For this review, use the dimensioned drawing (mm, ordinates from the lowest corner) and the shaded views. Round coordinates to 2 decimals unless told otherwise and drop trailing zeros. Order: outer loops, then holes, each group sorted by start corner. A loop starts at its lowest first (then second) coordinate and runs counter-clockwise, first axis right, second up. Notation, with made-up numbers: (-6, 13) -> (30, 13) arc R24 cw to (30, 49) -> close; hole circle Ø4 at (30.25, 27.25). An arc over 180 degrees is marked (long way). Use a Markdown table: item, result. Add a question column.
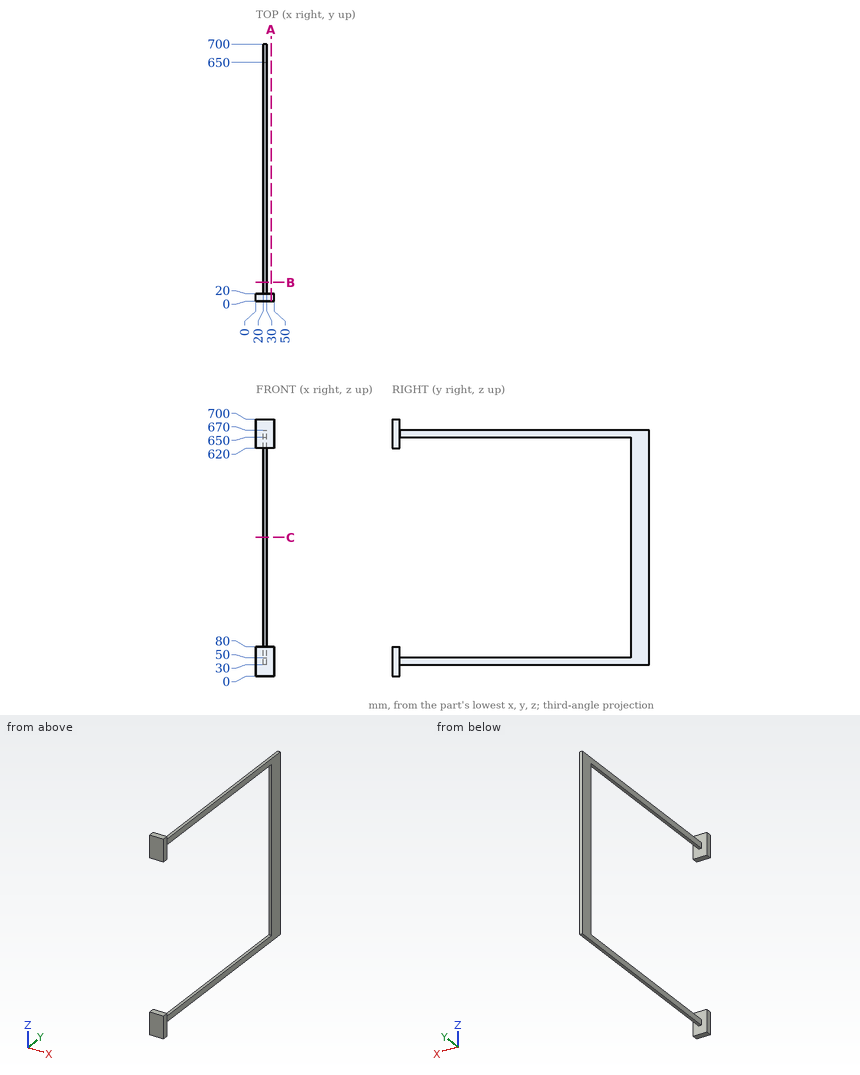
Q1. Add section A-A (x = 41.5). Write out the cut boundary in (y, z).
Q2. Add section C-C (z = 377.5). Write out the cut boundary in (x, y).
Q3. Wall thickness on line 1 (Z direction, x = 22, y = 443); line 2 (Y direction, x = 35, z = 657); line 3 (Y direction, x = 26.5, z = 180): over which ranges is each line inside the solid? List them lowest first. Write a range as [from, to].
Q4. Add section B-B (y = 50.5). Write out the cut boundary in (x, z), then the cut area to 3 significant figures.
Q5. Insertion check: pin 1 (8 mm diameter, centred on x = 26, y = 273, fed in from -Z); pin 2 (5 mm diameter, centred on x = 34, z = 367.5, fed in from -Y); pin 3 (11 mm diameter, centred on x = 26.5, z = 278, fed in from -Y); pin 4 (8 mm diameter, centred on x = 23.5, y = 275, fed in from +Z). Each pin has a flat end and moves straight along its axis. Give the tip position at first contact, or say it passes through.
Report:
| question | item | result |
|---|---|---|
| 1 | outline | (0, 0) -> (20, 0) -> (20, 80) -> (0, 80) -> close; (0, 620) -> (20, 620) -> (20, 700) -> (0, 700) -> close |
| 2 | outline | (20, 650) -> (30, 650) -> (30, 700) -> (20, 700) -> close |
| 3 | line 1 | z = [30, 50], [650, 670] |
| 3 | line 2 | y = [0, 20] |
| 3 | line 3 | y = [650, 700] |
| 4 | outline | (20, 30) -> (30, 30) -> (30, 50) -> (20, 50) -> close; (20, 650) -> (30, 650) -> (30, 670) -> (20, 670) -> close |
| 4 | area | 400 mm² |
| 5 | pin 1 | stops at z = 30 |
| 5 | pin 2 | passes through |
| 5 | pin 3 | stops at y = 650 |
| 5 | pin 4 | stops at z = 670 |
